The listing builds one solid part. Answer for the finished solid, in the listing's coordinates (mm). A direction names the side the tool comes from. Coordinates: 2 decimals unless noted, no trailing zeros. Order: outer loops, then holes, each group sorted by start corner. A loop starts at its lowest first (then second) coordinate and runs counter-clockwise, first axis right, second up. Notation, with made-up numbers: (66.5, 87) -> (74.5, 87) arc R20 ccw to (74.5, 123) -> close; hole circle Ø11 at (84, 26). An arc over 180 degrees is marked (long way). One line per question, with ' | ' between items.
from build123d import *

# Parameters (mm, degrees)
SKETCH3_R           = 1.5
BOSS_EXTRUDE1_DEPTH = 8
BOSS_EXTRUDE2_DEPTH = 8
BOSS_EXTRUDE3_DEPTH = 20
SKETCH10_R          = 7.5
SKETCH10_R_2        = 5
BOSS_EXTRUDE4_DEPTH = 10
FILLET1_R           = 3
CUT_EXTRUDE1_DEPTH  = 0.5
CUT_EXTRUDE2_START  = -0.5
CUT_EXTRUDE2_DEPTH  = 0.5
CHAMFER1_SIZE       = 3
SKETCH13_W          = 9.116659412
SKETCH13_H          = 8
BOSS_EXTRUDE5_DEPTH = 21
FILLET2_R           = 15
FILLET3_R           = 5
BOSS_EXTRUDE6_DEPTH = 7.5
SKETCH15_W          = 25
SKETCH15_H          = 10.000000005
CUT_EXTRUDE3_DEPTH  = 3
SKETCH17_W          = 25
SKETCH17_H          = 10.000000005
CUT_EXTRUDE4_DEPTH  = 3
FILLET4_R           = 3
SKETCH18_R          = 1.5
CUT_EXTRUDE5_DEPTH  = 36
SKETCH19_W          = 63.521473438
SKETCH19_H          = 44.294667312
CUT_EXTRUDE6_DEPTH  = 28.5
CHAMFER2_SIZE       = 1.5
FILLET5_R           = 1


with BuildPart() as part:
    # Sketch3 → Boss-Extrude1 (new body)
    with BuildSketch(Plane.XZ.offset(-5.496710387)):
        with BuildLine():
            Line((-58.572275019, 18.935598634), (-63.572275019, 18.935598634))
            Line((-63.572275019, 18.935598634), (-63.572275019, 5.639753178))
            Line((-63.572275019, 5.639753178), (-58.572275019, -7.656092278))
            Line((-58.572275019, -7.656092278), (-28.572248892, -7.656092278))
            Line((-28.572248892, -7.656092278), (-12.876703256, 8.039453359))
            Line((-12.876703256, 8.039453359), (-26.172535648, 21.335285751))
            Line((-26.172535648, 21.335285751), (-35.794074299, 11.7137471))
            ThreePointArc((-35.794074299, 11.7137471), (-43.572248892, 8.491921693), (-51.350423485, 11.7137471))
            Line((-51.350423485, 11.7137471), (-58.572275019, 18.935598634))
        make_face()
        with Locations((-33.672753955, -3.135495305)):
            Circle(SKETCH3_R, mode=Mode.SUBTRACT)
        with Locations((-20.944831894, 9.592426757)):
            Circle(SKETCH3_R, mode=Mode.SUBTRACT)
    extrude(amount=BOSS_EXTRUDE1_DEPTH)



with BuildPart() as body_2:
    # Sketch4 → Boss-Extrude2 (new body)
    with BuildSketch(Plane(origin=(0, 25.496710387, 0), x_dir=(1, 0, 0), z_dir=(0, 1, 0))):
        with BuildLine():
            Line((-65.072275019, -10.639753178), (-67.573393534, -10.639753178))
            Line((-67.573393534, -10.639753178), (-67.573393534, 7.656092278))
            Line((-67.573393534, 7.656092278), (-28.572248892, 7.656092278))
            Line((-28.572248892, 7.656092278), (-12.876703256, -8.039453359))
            Line((-12.876703256, -8.039453359), (-26.172535648, -21.335285751))
            Line((-26.172535648, -21.335285751), (-35.794074299, -11.7137471))
            ThreePointArc((-35.794074299, -11.7137471), (-43.572248892, -8.491921693), (-51.350423485, -11.7137471))
            Line((-51.350423485, -11.7137471), (-58.572275019, -18.935598634))
            Line((-58.572275019, -18.935598634), (-63.572275019, -18.935598634))
            Line((-63.572275019, -18.935598634), (-63.572275019, -12.139753178))
            ThreePointArc((-63.572275019, -12.139753178), (-64.011614847, -11.079093006), (-65.072275019, -10.639753178))
        make_face()
    extrude(amount=BOSS_EXTRUDE2_DEPTH)


with BuildPart() as part_1:
    add(part.part)

    add(body_2.part)  # Boss-Extrude3 merges body 2
    # Sketch9 → Boss-Extrude3 (add)
    with BuildSketch(Plane.XZ.offset(-25.496710387)):
        Polygon((-34.709554416, -7.656092278), (-42.709554416, 0.343907722), (-58.456734122, 0.343907722), (-58.456734122, -7.656092278), align=None)
    extrude(amount=BOSS_EXTRUDE3_DEPTH)

    # Sketch10 → Boss-Extrude4 (add)
    with BuildSketch(Plane(origin=(0, 0, -7.656092278), x_dir=(-1, 0, 0), z_dir=(0, 0, -1))):
        with Locations(Location((43.572275019, 15.496710387, 0), (0, 0, 180))):
            Circle(SKETCH10_R)
        with Locations((43.572275019, 15.496710387)):
            Circle(SKETCH10_R_2, mode=Mode.SUBTRACT)
    extrude(amount=BOSS_EXTRUDE4_DEPTH)

    # Fillet1
    fillet1_edges = [part_1.edges().sort_by_distance(p)[0] for p in [
        (-63.572275019, 1.496710387, 18.935598634),
        (-26.172535648, 1.496710387, 21.335285751),
        (-12.876703256, 1.496710387, 8.039453359),
        (-63.572275019, 29.496710387, 18.935598634),
        (-26.172535648, 29.496710387, 21.335285751),
        (-12.876703256, 29.496710387, 8.039453359),
    ]]
    fillet(fillet1_edges, radius=FILLET1_R)

    # Sketch11 → Cut-Extrude1 (cut)
    with BuildSketch(Plane.XZ.offset(-25.496710387)):
        with BuildLine():
            Line((-58.572275019, 18.935598634), (-60.572275019, 18.935598634))
            ThreePointArc((-60.572275019, 18.935598634), (-62.693595362, 18.056918977), (-63.572275019, 15.935598634))
            Line((-63.572275019, 15.935598634), (-63.572275019, 12.139753178))
            ThreePointArc((-63.572275019, 12.139753178), (-64.011614847, 11.079093006), (-65.072275019, 10.639753178))
            Line((-65.072275019, 10.639753178), (-67.573393534, 10.639753178))
            Line((-67.573393534, 10.639753178), (-67.573393534, -7.656092278))
            Line((-67.573393534, -7.656092278), (-58.456734122, -7.656092278))
            Line((-58.456734122, -7.656092278), (-58.456734122, 0.343907722))
            Line((-58.456734122, 0.343907722), (-42.709554416, 0.343907722))
            Line((-42.709554416, 0.343907722), (-34.709554416, -7.656092278))
            Line((-34.709554416, -7.656092278), (-28.572248892, -7.656092278))
            Line((-28.572248892, -7.656092278), (-14.998023599, 5.918133015))
            ThreePointArc((-14.998023599, 5.918133015), (-14.119343943, 8.039453359), (-14.998023599, 10.160773702))
            Line((-14.998023599, 10.160773702), (-24.051215304, 19.213965408))
            ThreePointArc((-24.051215304, 19.213965408), (-26.172535648, 20.092645064), (-28.293855992, 19.213965408))
            Line((-28.293855992, 19.213965408), (-35.794074299, 11.7137471))
            ThreePointArc((-35.794074299, 11.7137471), (-43.572248892, 8.491921693), (-51.350423485, 11.7137471))
            Line((-51.350423485, 11.7137471), (-58.572275019, 18.935598634))
        make_face()
    extrude(amount=-CUT_EXTRUDE1_DEPTH, mode=Mode.SUBTRACT)

    # Sketch12 → Cut-Extrude2 (cut)
    with BuildSketch(Plane(origin=(0, 5.496710387, 0), x_dir=(1, 0, 0), z_dir=(0, 1, 0)).offset(CUT_EXTRUDE2_START)):
        with BuildLine():
            Line((-67.573393534, -10.639753178), (-65.072275019, -10.639753178))
            ThreePointArc((-65.072275019, -10.639753178), (-64.011614847, -11.079093006), (-63.572275019, -12.139753178))
            Line((-63.572275019, -12.139753178), (-63.572275019, -15.935598634))
            ThreePointArc((-63.572275019, -15.935598634), (-62.693595362, -18.056918977), (-60.572275019, -18.935598634))
            Line((-60.572275019, -18.935598634), (-58.572275019, -18.935598634))
            Line((-58.572275019, -18.935598634), (-51.350423485, -11.7137471))
            ThreePointArc((-51.350423485, -11.7137471), (-43.572248892, -8.491921693), (-35.794074299, -11.7137471))
            Line((-35.794074299, -11.7137471), (-28.293855992, -19.213965408))
            ThreePointArc((-28.293855992, -19.213965408), (-26.172535648, -20.092645064), (-24.051215304, -19.213965408))
            Line((-24.051215304, -19.213965408), (-14.998023599, -10.160773702))
            ThreePointArc((-14.998023599, -10.160773702), (-14.119343943, -8.039453359), (-14.998023599, -5.918133015))
            Line((-14.998023599, -5.918133015), (-28.572248892, 7.656092278))
            Line((-28.572248892, 7.656092278), (-34.709554416, 7.656092278))
            Line((-34.709554416, 7.656092278), (-42.709554416, -0.343907722))
            Line((-42.709554416, -0.343907722), (-58.456734122, -0.343907722))
            Line((-58.456734122, -0.343907722), (-58.456734122, 7.656092278))
            Line((-58.456734122, 7.656092278), (-58.572275019, 7.656092278))
            Line((-58.572275019, 7.656092278), (-62.841209361, -3.695725977))
            ThreePointArc((-62.841209361, -3.695725977), (-63.941577707, -5.106321482), (-65.64921959, -5.639753178))
            Line((-65.64921959, -5.639753178), (-67.573393534, 7.656092278))
            Line((-67.573393534, 7.656092278), (-67.573393534, -10.639753178))
        make_face()
    extrude(amount=CUT_EXTRUDE2_DEPTH, mode=Mode.SUBTRACT)

    # Chamfer1
    # the kernel refuses this chamfer: 3 mm, written as the material it adds along each edge
    with BuildSketch(Plane(origin=(-43.572275019, 15.496710387, -7.656092278), x_dir=(1, 0, 0), z_dir=(0, 1, 0))) as chamfer1_piece_1_section:
        Polygon((7.5 + CHAMFER1_SIZE, 0), (7.5, CHAMFER1_SIZE), (7.5, 0), align=None)
    chamfer1_piece_1 = revolve(axis=Axis((-43.572275019, 15.496710387, -7.656092278), (0, 0, -1)), mode=Mode.PRIVATE)
    chamfer1_piece_1 = split(chamfer1_piece_1, bisect_by=Plane(origin=(-42.890914717, 15.496710387, 0.525268024), z_dir=(-0.7071067811865474, 0, -0.7071067811865477)), keep=Keep.TOP, mode=Mode.PRIVATE)
    add(chamfer1_piece_1)

    # Sketch13 → Boss-Extrude5 (add)
    with BuildSketch(Plane.XZ.offset(-25.996710387)):
        with Locations((-63.015063828, -3.656092278)):
            Rectangle(SKETCH13_W, SKETCH13_H)
    extrude(amount=BOSS_EXTRUDE5_DEPTH)

    # Fillet2
    fillet2_edges = [part_1.edges().sort_by_distance(p)[0] for p in [
        (-63.572275019, 1.246710387, 5.639753178),
    ]]
    fillet(fillet2_edges, radius=FILLET2_R)

    # Fillet3
    # the kernel refuses this fillet: 5 mm, written as the material it takes off along each edge
    with BuildSketch(Plane(origin=(-58.572275019, 20.819040858, 18.935598634), x_dir=(0.7071067811865416, 0, -0.7071067811865536), z_dir=(0, 1, 0)), Plane(origin=(-58.572275019, 10.174379917, 18.935598634), x_dir=(-1, 0, 0), z_dir=(0, -1, 0))) as fillet3_piece_1:
        with BuildLine():
            CenterArc((FILLET3_R * 0.414213562373, FILLET3_R), FILLET3_R, 225, 45)
            Line((-FILLET3_R * 0.292893218813, FILLET3_R * 0.292893218813), (-FILLET3_R * 0.307035354437, FILLET3_R * 0.27875108319))
            Line((-FILLET3_R * 0.307035354437, FILLET3_R * 0.27875108319), (-FILLET3_R * 0.00828427124746, -FILLET3_R * 0.02))
            Line((-FILLET3_R * 0.00828427124746, -FILLET3_R * 0.02), (FILLET3_R * 0.414213562373, -FILLET3_R * 0.02))
            Line((FILLET3_R * 0.414213562373, -FILLET3_R * 0.02), (FILLET3_R * 0.414213562373, 0))
        make_face()
    extrude(amount=17.855339059, mode=Mode.SUBTRACT)

    # Sketch14 → Boss-Extrude6 (add)
    with BuildSketch(Plane.XZ.offset(2.503289613)):
        with BuildLine():
            Line((-62.612326164, 3.087086856), (-58.572275019, -7.656092278))
            Line((-58.572275019, -7.656092278), (-67.573393534, -7.656092278))
            Line((-67.573393534, -7.656092278), (-67.573393534, 10.639753178))
            Line((-67.573393534, 10.639753178), (-65.072275019, 10.639753178))
            ThreePointArc((-65.072275019, 10.639753178), (-64.011614847, 11.079093006), (-63.572275019, 12.139753178))
            Line((-63.572275019, 12.139753178), (-63.572275019, 8.366950853))
            ThreePointArc((-63.572275019, 8.366950853), (-63.330336666, 5.683740759), (-62.612326164, 3.087086856))
        make_face()
    extrude(amount=-BOSS_EXTRUDE6_DEPTH)

    # Sketch15 → Cut-Extrude3 (cut)
    with BuildSketch(Plane.XZ.offset(2.503289613)):
        with Locations((-55.073393534, -2.656092276)):
            Rectangle(SKETCH15_W, SKETCH15_H)
    extrude(amount=-CUT_EXTRUDE3_DEPTH, mode=Mode.SUBTRACT)

    # Sketch17 → Cut-Extrude4 (cut)
    with BuildSketch(Plane(origin=(0, 33.496710387, 0), x_dir=(1, 0, 0), z_dir=(0, 1, 0))):
        with Locations((-55.073393534, 2.656092276)):
            Rectangle(SKETCH17_W, SKETCH17_H)
    extrude(amount=-CUT_EXTRUDE4_DEPTH, mode=Mode.SUBTRACT)

    # Fillet4
    fillet4_edges = [part_1.edges().sort_by_distance(p)[0] for p in [
        (-42.573393534, -1.003289613, 2.343907727),
        (-42.573393534, -1.003289613, -7.656092278),
        (-42.573393534, 31.996710387, 2.343907727),
        (-42.573393534, 31.996710387, -7.656092278),
    ]]
    fillet(fillet4_edges, radius=FILLET4_R)

    # Sketch18 → Cut-Extrude5 (cut)
    with BuildSketch(Plane.XZ.offset(2.503289613)):
        with Locations((-46.573393534, -3.65609228)):
            Circle(SKETCH18_R)
        with Locations((-63.573393534, -3.656092278)):
            Circle(SKETCH18_R)
    extrude(amount=-CUT_EXTRUDE5_DEPTH, mode=Mode.SUBTRACT)

    # Sketch19 → Cut-Extrude6 (cut)
    with BuildSketch(Plane(origin=(0, 33.496710387, 0), x_dir=(1, 0, 0), z_dir=(0, 1, 0))):
        with Locations((-40.836204684, -1.568816282)):
            Rectangle(SKETCH19_W, SKETCH19_H)
    extrude(amount=-CUT_EXTRUDE6_DEPTH, mode=Mode.SUBTRACT)

    # Chamfer2
    chamfer2_edges = [part_1.edges().sort_by_distance(p)[0] for p in [
        (-35.172753955, -2.503289613, -3.135495305),
        (-22.444831894, -2.503289613, 9.592426757),
    ]]
    chamfer(chamfer2_edges, length=CHAMFER2_SIZE)

    # Fillet5
    fillet5_edges = [part_1.edges().sort_by_distance(p)[0] for p in [
        (-67.573393534, 1.246710387, 10.639753178),
    ]]
    fillet(fillet5_edges, radius=FILLET5_R)


solid = part_1.part
Item 1: For faces 4 (the face through (-67.573, 2, 3)), 5 (the face through (-58.69, 1.3, 18.54)), 6 (the face through (-42.573, -1, -3)), determine the directions among +Z, -Z, +X, -X, +Y, -Y from which every point of the face is accessible in a straight line to the end or side of a thin tool.
Computed values:
face 4: +Z, -Z, -X, +Y, -Y | face 5: +Z, +Y, -Y | face 6: -Z, -X, -Y
Item 2: Find the intervals of material crossed by L1, parallel to X at y = 2, z = 9.5; L2, parallel to X at y = -1.5, z = 18; L3, parallel to Y at x = -60, z = -2.5, in increasing order.
Computed values:
L1: x = -67.57 to -48.17, -38.97 to -22.44, -19.45 to -14.5 | L2: x = -62.75 to -57.73, -29.51 to -22.84 | L3: y = 0.5 to 5
Item 3: Section A-A, the plane y = 1.75 is taken. Give the vertices of the cut face in (x, z), plus the area to 3 significant figures.
Computed values:
outline: (-67.57, -7.66) -> (-28.57, -7.66) -> (-15, 5.92) arc R3 ccw to (-15, 10.16) -> (-24.05, 19.21) arc R3 ccw to (-28.29, 19.21) -> (-35.79, 11.71) arc R11 cw to (-51.35, 11.71) -> (-57.11, 17.47) arc R5 ccw to (-60.6, 18.94) arc R3 ccw to (-63.57, 15.94) -> (-63.57, 12.14) arc R1.5 cw to (-65.07, 10.64) -> (-66.57, 10.64) arc R1 ccw to (-67.57, 9.64) -> close; hole circle Ø3 at (-63.57, -3.66); hole circle Ø3 at (-46.57, -3.66); hole circle Ø3 at (-33.67, -3.14); hole circle Ø3 at (-20.94, 9.59) | area: 1,010 mm^2
Item 4: Section B-B, the plane x = -50 is taken. Give the vertices of the cut face in (y, z).
Computed values:
outline: (-2.5, 2.34) -> (0.5, 2.34) -> (0.5, -7.66) -> (5, -7.66) -> (5, 10.57) -> (-2.5, 10.57) -> close
Item 5: Section C-C, the plane z = 0.5 is taken. Give the vertices of the cut face in (x, y).
Computed values:
outline: (-67.57, 0.5) -> (-42.81, 0.5) -> (-42.81, -2.5) -> (-20.42, -2.5) -> (-20.42, 5) -> (-67.57, 5) -> close
Item 6: Each of these flat-tipped pins is pushed along its axis until it touches: pin 1 Ø5 at (x, z) = (-47.5, -2.5) entering from -Y; pin 2 Ø2 at (x, y) = (-37.5, -1) entering from +Z; pin 3 Ø1.5 at (y, z) = (3.5, -4.5) entering from +X. Where does it stop, or does it pass through?
Computed values:
pin 1: stops at y = 0.5 | pin 2: stops at z = 11.07 | pin 3: stops at x = -24.67
Item 7: Determine the mould class of faces 1 (the face through (-45.14, 2.72, -3.21)), 2 (the face through (-54, 0.497, -3)), 3 (the face through (-66, 1, 10.64)) for opening direction Z: pulls with the +Z half, pulls with the -Z half, needs draft (parallel to the pull), parting line crosses it, or undercut.
Computed values:
face 1: undercut | face 2: needs draft | face 3: pulls with the +Z half
